Print and shaded views of the part. All mm, measured from the part's lowest x, y and z. Round coordinates to 2 decimals unless told otherwise and drop trailing zeros. Loops run counter-clockwise (first coordinate to the right, second up) from the corner with the lowest first, then second, coordinate; pieces in that order, holes last. Notation, with made-up numbers: (-11, -14.5) -> (42, -14.5) arc R27 cw to (42, 23.5) -> close; hole circle Ø10 at (-12, 54.25). An arc over 180 degrees is marked (long way). Use a Markdown table: item, result.
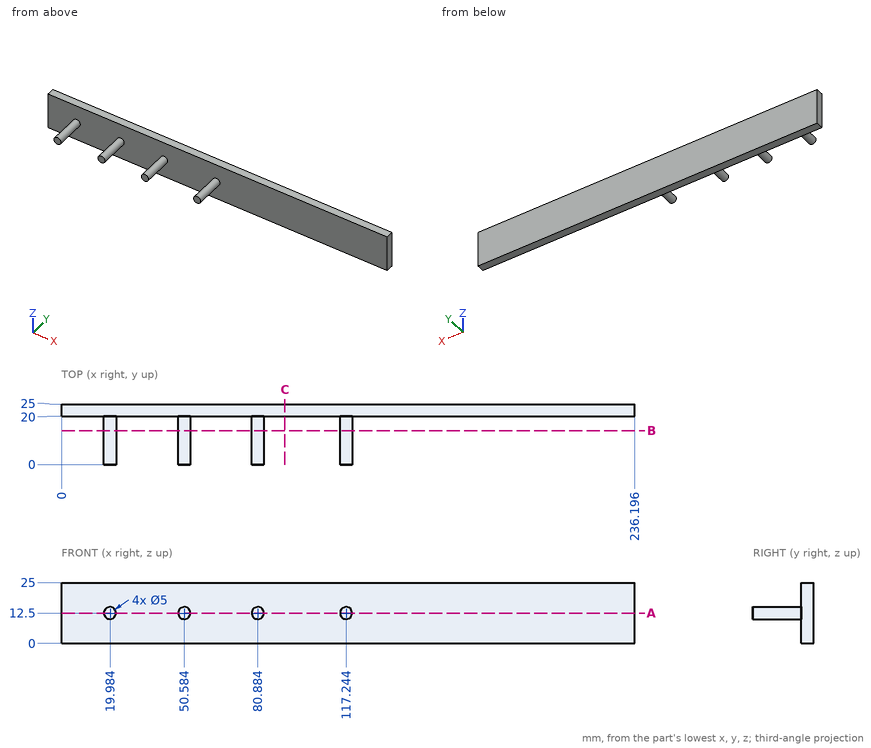
Q1. Band-saw the part on C-C, the plane x = 92. Give the cut face in (y, z).
Results list:
| item | result |
|---|---|
| outline | (20, 0) -> (25, 0) -> (25, 25) -> (20, 25) -> close |
Q2. Flat gauge pins, fed straight in: pin 1 (4 mm diameter, centred on x = 149.5, z = 14.5, fed in from -Y); pin 2 (4 mm diameter, centred on y = 9, z = 15, fed in from +X). Where does each tip first touch, or does it go through?
Results list:
| item | result |
|---|---|
| pin 1 | stops at y = 20 |
| pin 2 | stops at x = 119.69 |
Q3. Band-saw the part on A-A, the plane z = 12.5. Give the cut face in (x, y), plus the area to 3 significant figures.
Results list:
| item | result |
|---|---|
| outline | (0, 20) -> (17.48, 20) -> (17.48, 0) -> (22.48, 0) -> (22.48, 20) -> (48.08, 20) -> (48.08, 0) -> (53.08, 0) -> (53.08, 20) -> (78.38, 20) -> (78.38, 0) -> (83.38, 0) -> (83.38, 20) -> (114.74, 20) -> (114.74, 0) -> (119.74, 0) -> (119.74, 20) -> (236.2, 20) -> (236.2, 25) -> (0, 25) -> close |
| area | 1,580 mm² |
Q4. Band-saw the part on B-B, the plane y = 14. Give the cut face in (x, z).
Results list:
| item | result |
|---|---|
| outline | circle Ø5 at (19.98, 12.5); circle Ø5 at (50.58, 12.5); circle Ø5 at (80.88, 12.5); circle Ø5 at (117.24, 12.5) |
Q5. Drill centre lines: L1, parallel to X at y = 9, z = 14 (1 decimal); L2, parallel to X at y = 2.5, z = 11.25; L3, parallel to Y at x = 188, z = 1.75. Where is each one in solid material? Low to high. Write a range as from..to.
Results list:
| item | result |
|---|---|
| L1 | x = 18..22, 48.6..52.6, 78.9..82.9, 115.2..119.2 |
| L2 | x = 17.82..22.15, 48.42..52.75, 78.72..83.05, 115.08..119.41 |
| L3 | y = 20..25 |
